Build history of the part. All positions in model axes, mm. A direction names the side the tool comes from. Give positions to 0.01 mm unless a question says otherwise; leave off trailing zeros. Loops run counter-clockwise (first coordinate to the right, second up) from the corner with the lowest first, then second, coordinate; pieces in that order, holes last. Notation, with made-up numbers: M -37,0.5 L -9,0.5 A26 cw -9,19.5 Z; hole C 32,5.5 d7. An arc over 180 degrees is marked long. Put each result on its own line as item: value.
```python
from build123d import *

# Parameters (mm, degrees)
F0_W     = 24
F0_H     = 10
F1_DEPTH = 24
F2_W     = 24
F2_H     = 5
F3_DEPTH = 8
F5_DEPTH = 24.001
F7_DEPTH = 10
F8_W     = 10.2
F8_H     = 2
F9_DEPTH = 6
F10_SIZE = 1


with BuildPart() as f1:
    # F0 (on Front) → F1 (new body)
    with BuildSketch(Plane.XZ):
        Rectangle(F0_W, F0_H)
    extrude(amount=F1_DEPTH)

    # F2 (on face) → F3 (cut)
    with BuildSketch(Plane.XZ.offset(24)):
        with Locations((0, -2.5)):
            Rectangle(F2_W, F2_H)
    extrude(amount=-F3_DEPTH, mode=Mode.SUBTRACT)

    # F4 (on face) → F5 (cut, through all)
    with BuildSketch(Plane(origin=(0, 0, 0), x_dir=(-1, 0, 0), z_dir=(0, 1, 0))):
        with BuildLine():
            Line((-1.8, -5), (1.8, -5))
            add(Edge.make_bspline(
                [(1.8, -5), (1.8, -3.05), (0, -3.05), (-1.8, -3.05), (-1.8, -5)],
                knots=[4.7123889804, 4.7123889804, 4.7123889804, 6.2831853072, 6.2831853072, 7.853981634, 7.853981634, 7.853981634], degree=2, weights=[1, 0.7071067812, 1, 0.7071067812, 1]))
        make_face()
    extrude(amount=-F5_DEPTH, mode=Mode.SUBTRACT)

    # F6 (on face) → F7 (cut)
    with BuildSketch(Plane(origin=(0, 0, 0), x_dir=(-1, 0, 0), z_dir=(0, 1, 0))):
        Polygon((-1.8, -5), (1.8, -5), (12, -5), (12, 0), (-12, 0), (-12, -5), align=None)
    extrude(amount=-F7_DEPTH, mode=Mode.SUBTRACT)

    # F8 (on face) → F9 (join, through all)
    with BuildSketch(Plane.XZ.offset(16)):
        with Locations((-6.9, -6)):
            Rectangle(F8_W, F8_H)
        with Locations((6.9, -6)):
            Rectangle(F8_W, F8_H)
    extrude(amount=-F9_DEPTH)

    # F10
    f10_edges = [f1.edges().sort_by_distance(p)[0] for p in [
        (-1.8, -13, -7),
        (1.8, -13, -7),
    ]]
    chamfer(f10_edges, length=F10_SIZE)


solid = f1.part
```
Q1. Slice it at C-C (y = -7.25). List the corners of the cut face in (x, z), and give its area (3 significant figures).
Here are the results:
outline: M -12,0 L 12,0 L 12,5 L -12,5 Z
area: 120 mm²
Q2. Probe line 1 (Z direction, x = 6, y = -0.75); line 2 (Y direction, x = -9.25, z = -1); line 3 (X direction, y = -10.75, z = -3.5). List the from-to ranges inside material, lowest first. Write a range as from..to.
Here are the results:
line 1: 0..5
line 2: -16..-10
line 3: -12..-1.15, 1.15..12
Q3. Slice it at A-A (z = -5.5). List the corners of the cut face in (x, y), and give its area (3 significant figures).
Here are the results:
outline: M -12,-16 L -1.8,-16 L -1.8,-10 L -12,-10 Z; M 1.8,-16 L 12,-16 L 12,-10 L 1.8,-10 Z
area: 122 mm²
Q4. Mould opens along X. For faces 4 (the flat face through (-12, -12, 2)), 5 (the flat face through (0, 0, 3)), 6 (the flat face through (12, -12, 2)), 7 (the flat face through (1.8, -13, -5.5)) say: pulls with the +X half, pulls with the -X half, needs draft (parallel to the pull), parting line crosses it, or undercut.
Here are the results:
face 4: pulls with the -X half
face 5: needs draft
face 6: pulls with the +X half
face 7: undercut
Q5. Drop flat-ended pins along their axis: pin 1 Ø4 at (x, y) = (-4.5, -19) entering from -Z; pin 2 Ø3 at (x, z) = (2, -4) entering from -Y; pin 3 Ø5.5 at (x, z) = (5.5, -3.5) entering from +Y. Give the stop position or say it passes through.
Here are the results:
pin 1: z = 0
pin 2: y = -16
pin 3: y = -10
Q6. Tool access for faces 1 (the flat face through (-2.3, -13, -6.5)), 2 (the flat face through (0, -5, 0)), 3 (the flat face through (0, -20, 0)): list every direction of +Z, -Z, +X, -X, +Y, -Y with a clear straight run to the whole face (end or side of a thin tool).
Here are the results:
face 1: -Z, +Y, -Y
face 2: -Z, +X, -X, +Y
face 3: -Z, +X, -X, -Y
Q7. Slice it at B-B (x = -6). List the corners of the cut face in (y, z), and give its area (3 significant figures).
Here are the results:
outline: M -24,0 L -16,0 L -16,-7 L -10,-7 L -10,0 L 0,0 L 0,5 L -24,5 Z
area: 162 mm²
